Part model, mm, in its own coordinate system. A direction names the side the tool comes from. Coordinates: 2 decimals unless noted, no trailing zeros. Loops run counter-clockwise (first coordinate to the right, second up) from the corner with the lowest first, then second, coordinate; pieces in that order, holes last. Notation, with made-up numbers: M 61.5,-9 L 94.5,-9 A22 ccw 94.5,29 Z; hole C -15.75,78.5 d6. An arc over 180 degrees is marked long. Answer as a JSON object with one key per item and string values. Group by question number.
1. Saw through at B-B on z = -4. Write the cut outline in (x, y), then the cut area to 3 significant figures.
2. Saw through at A-A on z = 13.5. Write the cut outline in (x, y) (3 decimals).
3. Drop a flat-ended pin along its axis: pin 1 Ø1.5 at (x, y) = (-2.5, 1.5) entering from +Z. Give the stop position or say it passes through.
4. Drill centre lines: L1, parallel to Z at x = 1, y = 0; L2, parallel to X at y = 1, z = -4.5; L3, parallel to X at y = -0.5, z = 5.75. Where is each one in solid material? Low to high.
5. 3-axis set-ups, long thin cutter, end or side, ignore diameter. For faces 1 (the face through (0, 1, 0)), 2 (the face through (1.5, -0.07, -8.58)), 3 (the face through (-3.047, -0.134, -3.783)): which of +Z, -Z, +X, -X, +Y, -Y reach the whole face in a straight line?
Autodesk Inventor part; units mm, degrees
ref_plane "YZ Plane" through (0, 0, 0) normal (1, 0, 0) x (0, 1, 0)
ref_plane "XZ Plane" through (0, 0, 0) normal (0, 1, 0) x (-1, 0, 0)
ref_plane "XY Plane" through (0, 0, 0) normal (0, 0, 1) x (1, 0, 0)
sketch "Sketch1" plane through (0, 0, 0) normal (0, 1, 0) x (-1, 0, 0)
  line L0 (0, 0) -> (-3.05, 0)
  line L1 (-3.05, 0) -> (-3.05, -6.604)
  line L2 (-3.05, -6.604) -> (0, -6.604)
  line L3 (0, -6.604) -> (0, 0)
  line L4 (0, 0) -> (-0.635, 0)
  line L5 (-0.635, 0) -> (-0.635, 14.605)
  line L6 (-0.635, 14.605) -> (0, 14.605)
  line L7 (0, 14.605) -> (0, 0)
  line L8 (-0.635, 14.605) -> (0, 16.9749)
  line L9 (-0.635, 14.605) -> (1.8185, 14.605) construction
  line L10 (0, 16.9749) -> (0, 14.605)
  dimension "d0" = 3.05
  dimension "d1" = 6.604
  dimension "d2" = 0.635
  dimension "d3" = 14.605
  dimension "d13" = 75
  dimension "d14" = 15
  dimension "d15" = 16.9748
  dimension "d16" = 23.5788
revolve "Revolution1" add sketch "Sketch1" angle 360 about axis through (0, 0, 14.605) along (0, 0, -1)
sketch "Sketch2" plane through (0, 0, -6.604) normal (0, 0, -1) x (-1, 0, 0)
  circle A0 centre (0, 0) radius 3.05
  circle A1 centre (0, 0) radius 1.5
  dimension "d5" = 3
extrude "Extrusion1" add sketch "Sketch2" along normal blind 4 contours A1
chamfer "Chamfer1" distance 1.143 angle 45 1 edges at (-3.05, 0, 0)
chamfer "Chamfer2" distance 0.254 angle 45 1 edges at (-3.05, 0, -6.604)
thread "Thread1"
properties part number "carbide_probe_30deg_tip_r02" material "Steel, High Strength, Low Alloy"
Outcome:
{
 "1": {"outline": "C 0,0 d6.1", "area": "29.2 mm²"},
 "2": {"outline": "C 0,0 d1.27"},
 "3": {"pin 1": "stops at z = -0.26"},
 "4": {"L1": "z = -10.6 to 0", "L2": "x = -2.88 to 2.88", "L3": "x = -0.39 to 0.39"},
 "5": {"face 1": "+Z", "face 2": "-Z", "face 3": "+Z, -Z"}
}
